from build123d import *

# Parameters (mm, degrees)
SKETCH1_R           = 9.5
SKETCH1_R_2         = 3
BOSS_EXTRUDE1_DEPTH = 6
SKETCH2_R           = 8
SKETCH2_R_2         = 5.5
CUT_EXTRUDE1_DEPTH  = 0.2
SKETCH3_R           = 8
SKETCH3_R_2         = 5.5
CUT_EXTRUDE2_DEPTH  = 0.2
CHAMFER1_SIZE       = 0.2


with BuildPart() as part:
    # Sketch1 → Boss-Extrude1 (new body)
    with BuildSketch(Plane(origin=(0, 0, 0), x_dir=(1, 0, 0), z_dir=(0, 1, 0))):
        Circle(SKETCH1_R)
        Circle(SKETCH1_R_2, mode=Mode.SUBTRACT)
    extrude(amount=BOSS_EXTRUDE1_DEPTH)

    # Sketch2 → Cut-Extrude1 (cut)
    with BuildSketch(Plane(origin=(0, 6, 0), x_dir=(1, 0, 0), z_dir=(0, 1, 0))):
        Circle(SKETCH2_R)
        Circle(SKETCH2_R_2, mode=Mode.SUBTRACT)
    extrude(amount=-CUT_EXTRUDE1_DEPTH, mode=Mode.SUBTRACT)

    # Sketch3 → Cut-Extrude2 (cut)
    with BuildSketch(Plane.XZ):
        Circle(SKETCH3_R)
        Circle(SKETCH3_R_2, mode=Mode.SUBTRACT)
    extrude(amount=-CUT_EXTRUDE2_DEPTH, mode=Mode.SUBTRACT)

    # Chamfer1
    chamfer1_edges = [part.edges().sort_by_distance(p)[0] for p in [
        (-9.5, 0, 0),
        (-9.5, 6, 0),
        (-3, 0, 0),
        (-3, 6, 0),
    ]]
    chamfer(chamfer1_edges, length=CHAMFER1_SIZE)


solid = part.part
Work out the finished part from the listing and answer in its coordinate system (mm). Coordinates: 2 decimals unless noted, no trailing zeros. Loops run counter-clockwise (first coordinate to the right, second up) from the corner with the lowest first, then second, coordinate; pieces in that order, holes last. Notation, with made-up numbers: M 85.25,63 L 144.25,63 A25 cw 144.25,101 Z; hole C -24.75,-6 d7. An arc over 180 degrees is marked long. Answer in a Markdown table with one row per item. Add a question column.
1. Find section C-C, the plane y = 3.6. Write down the section's boundary in (x, z).
2. The mould has two halves that part along X. Classify faces 1 (the cylindrical face through (4.38, 2.96, 8.43)), 2 (the flat face through (1.7, 5.8, -5.4)), 3 (the flat face through (3, 0, -8)), 4 (the flat face through (1.7, 0.2, 5.4)): pulls with the +X half, pulls with the -X half, needs draft (parallel to the pull), parting line crosses it, or undercut.
3. Consider L1, parallel to Z at x = 0, y = 2.65; L2, parallel to Z at x = 0, y = 0.1. Determine where each line is inside the solid, lowest interval first.
4. Flat-ended cylindrical pins translate along their axes: P1, Ø1, axis at x = -1.5, y = 5, coming from the -Z side; P2, Ø3, axis at x = 7.5, z = 1, coming from the +Y side. Find the tip coordinate at first contact, or state that the pin passes through.
Reported:
| question | item | result |
|---|---|---|
| 1 | outline | C 0,0 d19; hole C 0,0 d6 |
| 2 | face 1 | parting line crosses it |
| 2 | face 2 | undercut |
| 2 | face 3 | needs draft |
| 2 | face 4 | undercut |
| 3 | L1 | z = -9.5 to -3, 3 to 9.5 |
| 3 | L2 | z = -9.4 to -8, -5.5 to -3.1, 3.1 to 5.5, 8 to 9.4 |
| 4 | P1 | stops at z = -9.45 |
| 4 | P2 | stops at y = 6 |
